Source: CAD feature listing. Evaluate the final solid. Frame: model axes, mm. Coordinates: 2 decimals unless noted, no trailing zeros. Write each loop counter-clockwise with the first axis right and the second up, starting at its lowest first coordinate (ties: lowest second). Pieces come first, ordered by that corner, then holes. Notation, with made-up numbers: M 69.25,52.5 L 97.25,52.5 A24 ccw 97.25,62.5 Z; hole C 76,58 d5. An arc over 180 degrees is marked long. Answer as CSV lines item,"result". Start each with the question number.
1. Section B-B on z = 64. Return the cut outline in (x, y), plus the area to 3 significant figures.
2. Section C-C on z = 99.5. Return the cut outline in (x, y).
3. Contact query for flat-ended pins moving along their axis: pin 1 Ø1.9 at (x, y) = (-4.5, -4) entering from -Z; pin 2 Ø3 at (y, z) = (-4, 27) entering from -X; pin 3 Ø1 at (x, y) = (35, -4.5) entering from +Z; pin 4 Ø3.5 at (x, z) = (6.15, 16.15) entering from +Y. Output: stop coordinate, or through.
4. Section D-D on y = -1. Count the separate pieces of the cut face and the enclosed holes in it, plus the area to 3 significant figures.
5. Line query: probe 1 along Z at (x, y) = (13.65, -2.5) (3 decimals); probe 2 along X at (y, z) = (-1.75, 121.15); probe 3 along Z at (x, y) = (161.15, -3.75). Output: solid intervals per line, ascending. Write a range as [from, to].
6. Section A-A on x = 81. Return the cut outline in (y, z), plus the area to 3 significant figures.
```python
from build123d import *

# Parameters (mm, degrees)
F0_R     = 1.5
F1_DEPTH = 6.35


with BuildPart() as f1:
    # F0 (on Front) → F1 (new body)
    with BuildSketch(Plane.XZ):
        with BuildLine():
            Line((0, 15), (0, 0))
            Line((0, 0), (8.65, 0))
            Line((8.65, 0), (8.65, -6.35))
            ThreePointArc((8.65, -6.35), (13.65, -7.689746), (18.65, -6.35))
            Line((18.65, -6.35), (18.65, 0))
            Line((18.65, 0), (148.65, 0))
            Line((148.65, 0), (148.65, -6.35))
            ThreePointArc((148.65, -6.35), (153.65, -7.689746), (158.65, -6.35))
            Line((158.65, -6.35), (158.65, -6.289838))
            Line((158.65, -6.289838), (158.65, 0))
            Line((158.65, 0), (167.3, 0))
            Line((167.3, 0), (167.3, 15))
            Line((167.3, 15), (173.65, 15))
            ThreePointArc((173.65, 15), (174.989746, 20), (173.65, 25))
            Line((173.65, 25), (167.3, 25))
            Line((167.3, 25), (167.3, 102.3))
            Line((167.3, 102.3), (173.65, 102.3))
            ThreePointArc((173.65, 102.3), (174.989746, 107.3), (173.65, 112.3))
            Line((173.65, 112.3), (167.3, 112.3))
            Line((167.3, 112.3), (167.3, 127.3))
            Line((167.3, 127.3), (158.65, 127.3))
            Line((158.65, 127.3), (158.65, 133.65))
            ThreePointArc((158.65, 133.65), (153.65, 134.989746), (148.65, 133.65))
            Line((148.65, 133.65), (148.65, 127.3))
            Line((148.65, 127.3), (18.65, 127.3))
            Line((18.65, 127.3), (18.65, 133.65))
            ThreePointArc((18.65, 133.65), (13.65, 134.989746), (8.65, 133.65))
            Line((8.65, 133.65), (8.65, 127.3))
            Line((8.65, 127.3), (0, 127.3))
            Line((0, 127.3), (0, 112.3))
            Line((0, 112.3), (-6.35, 112.3))
            ThreePointArc((-6.35, 112.3), (-7.689746, 107.3), (-6.35, 102.3))
            Line((-6.35, 102.3), (0, 102.3))
            Line((0, 102.3), (0, 25))
            Line((0, 25), (-6.35, 25))
            ThreePointArc((-6.35, 25), (-7.689746, 20), (-6.35, 15))
            Line((-6.35, 15), (0, 15))
        make_face()
        with Locations((13.65, -3.175)):
            Circle(F0_R, mode=Mode.SUBTRACT)
        with Locations((6.15, 16.15)):
            Circle(F0_R, mode=Mode.SUBTRACT)
        with Locations((-3.175, 20)):
            Circle(F0_R, mode=Mode.SUBTRACT)
        with BuildLine():
            Line((32.471991, 25.806455), (134.828009, 25.806455))
            ThreePointArc((134.828009, 25.806455), (130.075832, 20.107324), (124.692661, 15))
            Line((124.692661, 15), (42.607339, 15))
            ThreePointArc((42.607339, 15), (37.224168, 20.107324), (32.471991, 25.806455))
        make_face(mode=Mode.SUBTRACT)
        with BuildLine():
            Line((22.104172, 47.419365), (145.195828, 47.419365))
            ThreePointArc((145.195828, 47.419365), (143.478503, 41.927369), (141.272203, 36.61291))
            Line((141.272203, 36.61291), (26.027797, 36.61291))
            ThreePointArc((26.027797, 36.61291), (23.821497, 41.927369), (22.104172, 47.419365))
        make_face(mode=Mode.SUBTRACT)
        with Locations((153.65, -3.175)):
            Circle(F0_R, mode=Mode.SUBTRACT)
        with Locations((161.15, 16.15)):
            Circle(F0_R, mode=Mode.SUBTRACT)
        with Locations((170.475, 20)):
            Circle(F0_R, mode=Mode.SUBTRACT)
        with BuildLine():
            ThreePointArc((20.1014, 60.058627), (20.006631, 64.568711), (20.231542, 69.074179))
            Line((20.231542, 69.074179), (147.068458, 69.074179))
            ThreePointArc((147.068458, 69.074179), (147.299997, 63.671028), (147.072028, 58.267724))
            Line((147.072028, 58.267724), (20.227972, 58.267724))
            ThreePointArc((20.227972, 58.267724), (20.158371, 59.162729), (20.1014, 60.058627))
        make_face(mode=Mode.SUBTRACT)
        with BuildLine():
            ThreePointArc((22.104172, 79.880635), (23.821497, 85.372631), (26.027797, 90.68709))
            Line((26.027797, 90.68709), (141.272203, 90.68709))
            ThreePointArc((141.272203, 90.68709), (143.478503, 85.372631), (145.195828, 79.880635))
            Line((145.195828, 79.880635), (22.104172, 79.880635))
        make_face(mode=Mode.SUBTRACT)
        with Locations((-3.175, 107.3)):
            Circle(F0_R, mode=Mode.SUBTRACT)
        with Locations((6.15, 121.15)):
            Circle(F0_R, mode=Mode.SUBTRACT)
        with Locations((13.65, 130.475)):
            Circle(F0_R, mode=Mode.SUBTRACT)
        with BuildLine():
            ThreePointArc((32.471991, 101.493545), (37.224168, 107.192676), (42.607339, 112.3))
            Line((42.607339, 112.3), (124.692661, 112.3))
            ThreePointArc((124.692661, 112.3), (130.075832, 107.192676), (134.828009, 101.493545))
            Line((134.828009, 101.493545), (32.471991, 101.493545))
        make_face(mode=Mode.SUBTRACT)
        with Locations((170.475, 107.3)):
            Circle(F0_R, mode=Mode.SUBTRACT)
        with Locations((161.15, 121.15)):
            Circle(F0_R, mode=Mode.SUBTRACT)
        with Locations((153.65, 130.475)):
            Circle(F0_R, mode=Mode.SUBTRACT)
    extrude(amount=F1_DEPTH)


solid = f1.part
```
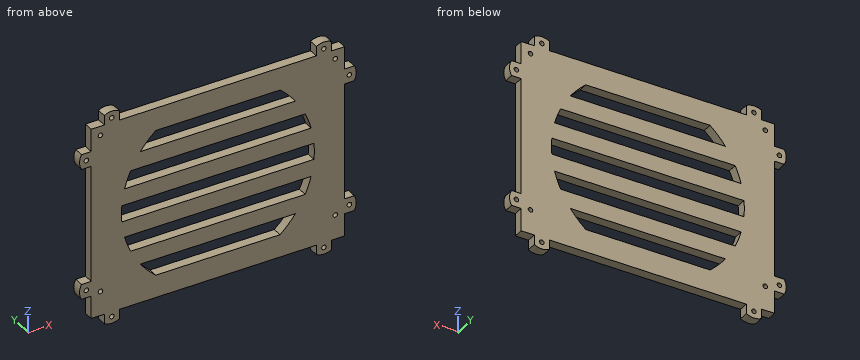
Values:
1,outline,"M 0,-6.35 L 20,-6.35 L 20,0 L 0,0 Z; M 147.3,-6.35 L 167.3,-6.35 L 167.3,0 L 147.3,0 Z"
1,area,"254 mm²"
2,outline,"M 0,-6.35 L 167.3,-6.35 L 167.3,0 L 0,0 Z"
3,pin 1,"z = 15"
3,pin 2,"x = 0"
3,pin 3,"z = 127.3"
3,pin 4,"y = 0"
4,separate pieces,"1"
4,enclosed holes,"17"
4,area,"15,800 mm²"
5,probe 1,"[-7.69, -4.675], [-1.675, 128.975], [131.975, 134.99]"
5,probe 2,"[0, 4.65], [7.65, 159.65], [162.65, 167.3]"
5,probe 3,"[0, 14.65], [17.65, 119.65], [122.65, 127.3]"
6,outline,"M -6.35,0 L 0,0 L 0,15 L -6.35,15 Z; M -6.35,25.81 L 0,25.81 L 0,36.61 L -6.35,36.61 Z; M -6.35,47.42 L 0,47.42 L 0,58.27 L -6.35,58.27 Z; M -6.35,69.07 L 0,69.07 L 0,79.88 L -6.35,79.88 Z; M -6.35,90.69 L 0,90.69 L 0,101.49 L -6.35,101.49 Z; M -6.35,112.3 L 0,112.3 L 0,127.3 L -6.35,127.3 Z"
6,area,"465 mm²"
